```python
from build123d import *

# Parameters (mm, degrees)
F1_DEPTH = 10
F2_R     = 2.6409813422
F2_R_2   = 2.1665688489
F3_DEPTH = 1


# Not quite as in the source:
# - a feature names something its author has since deleted; it is built from what else it names


with BuildPart() as f1:
    # F0 (on Front) → F1 (new body)
    with BuildSketch(Plane.XZ):
        Polygon((-49.4838858729, 98.9949493661), (-56.5549536848, 91.9238815543), (42.4399956814, -7.0710678119), (49.5110634932, 0), align=None)
    extrude(amount=F1_DEPTH)

    # F2 (on face) → F3 (join)
    with BuildSketch(Plane.XZ.offset(10)):
        with Locations((41.9252365828, 0)):
            Circle(F2_R)
        with Locations((-48.3359694481, 91.1623910069)):
            Circle(F2_R_2)
    extrude(amount=F3_DEPTH)


solid = f1.part
```
Input: part model. Units: mm. Frame: model coordinates. A direction names the side the tool comes from. Coordinates: 2 decimals unless noted, no trailing zeros. Loops run counter-clockwise (first coordinate to the right, second up) from the corner with the lowest first, then second, coordinate; pieces in that order, holes last. Notation, with made-up numbers: (-31, -28) -> (27, -28) arc R27 ccw to (27, -10) -> close; hole circle Ø3 at (77.5, 44). An arc over 180 degrees is marked (long way). Use a Markdown table: item, result.
1) Cut plane B-B (z = 32). Return the cut outline in (x, y).
Results found:
| item | result |
|---|---|
| outline | (3.37, -10) -> (17.51, -10) -> (17.51, 0) -> (3.37, 0) -> close |
2) Access query for faces 1 (the cylindrical face through (-48.62, -10.49, 93.31)), 2 (the flat face through (42, -11, 0)). Directions: +Z, -Z, +X, -X, +Y, -Y. A direction counts if a zero-diameter tool reaches every point of the face in a straight line with its end or side. Return the directions, or none.
Results found:
| item | result |
|---|---|
| face 1 | -Y |
| face 2 | +Z, -Z, +X, -X, -Y |
3) Contact query for flat-ended pins moving along their axis: pin 1 (3 mm diameter, centred on x = 20, z = 17, fed in from -Y); pin 2 (3 mm diameter, centred on y = -5, z = 72.5, fed in from -X); pin 3 (2 mm diameter, centred on x = -9, y = -3.5, fed in from +Z). Output: stop coordinate, or through.
Results found:
| item | result |
|---|---|
| pin 1 | stops at y = -10 |
| pin 2 | stops at x = -38.63 |
| pin 3 | stops at z = 59.51 |
4) Cut plane A-A (y = -2). Return the cut outline in (x, z), then the cut area to 3 significant figures.
Results found:
| item | result |
|---|---|
| outline | (-56.55, 91.92) -> (42.44, -7.07) -> (49.51, 0) -> (-49.48, 98.99) -> close |
| area | 1,400 mm2 |
5) Material intervals for line 1 along Y through (x, z) = (-45.5, 87.5); line 2 along Z through (x, y) = (45.5, -9.75); line 3 along X through (y, z) = (-9, 88), sorted ascending. Write a range as from..to.
Results found:
| item | result |
|---|---|
| line 1 | y = -10..0 |
| line 2 | z = -4.01..4.01 |
| line 3 | x = -52.63..-38.49 |
